Autodesk Inventor part; units mm, degrees
ref_plane "Work Plane1" through (0, 0, 0) normal (0, 0, 1) x (1, 0, 0)
ref_plane "YZ Plane" through (0, 0, 0) normal (1, 0, 0) x (0, 1, 0)
ref_plane "XZ Plane" through (0, 0, 0) normal (0, 1, 0) x (-1, 0, 0)
ref_plane "Work Plane1" through (0, 0, 0) normal (0, 0, 1) x (1, 0, 0)
sketch "Sketch1" plane through (0, 0, 0) normal (0, 0, 1) x (1, 0, 0)
  arc A0 (535, 222.5775) -> (565, 252.5775) centre (535, 252.5775) ccw
  line L0 (535, 222.5775) -> (295, 222.5775)
  arc A1 (265, 252.5775) -> (295, 222.5775) centre (295, 252.5775) ccw
  line L1 (265, 252.5775) -> (265, 402.5775)
  arc A2 (295, 432.5775) -> (265, 402.5775) centre (295, 402.5775) ccw
  line L2 (295, 432.5775) -> (535, 432.5775)
  arc A3 (565, 402.5775) -> (535, 432.5775) centre (535, 402.5775) ccw
  line L3 (565, 402.5775) -> (565, 252.5775)
  arc A4 (535, -104.9225) -> (565, -74.9225) centre (535, -74.9225) ccw
  line L4 (535, -104.9225) -> (295, -104.9225)
  arc A5 (265, -74.9225) -> (295, -104.9225) centre (295, -74.9225) ccw
  line L5 (265, -74.9225) -> (265, 75.0775)
  arc A6 (295, 105.0775) -> (265, 75.0775) centre (295, 75.0775) ccw
  line L6 (295, 105.0775) -> (535, 105.0775)
  arc A7 (565, 75.0775) -> (535, 105.0775) centre (535, 75.0775) ccw
  line L7 (565, 75.0775) -> (565, -74.9225)
  line L8 (565, -252.4225) -> (565, -402.4225)
  arc A8 (535, -432.4225) -> (565, -402.4225) centre (535, -402.4225) ccw
  line L9 (535, -432.4225) -> (295, -432.4225)
  arc A9 (265, -402.4225) -> (295, -432.4225) centre (295, -402.4225) ccw
  line L10 (265, -402.4225) -> (265, -252.4225)
  arc A10 (295, -222.4225) -> (265, -252.4225) centre (295, -252.4225) ccw
  line L11 (295, -222.4225) -> (535, -222.4225)
  arc A11 (565, -252.4225) -> (535, -222.4225) centre (535, -252.4225) ccw
  line L12 (-550, 375.7749) -> (-550, 187.5)
  arc A12 (-473.6326, 455.6923) -> (-550, 375.7749) centre (-470, 375.7749) ccw
  line L13 (229.0918, 487.6344) -> (-473.6326, 455.6923)
  arc A13 (250, 467.655) -> (229.0918, 487.6344) centre (230, 467.655) ccw
  line L14 (250, 187.5) -> (250, 467.655)
  arc A14 (230, 167.5) -> (250, 187.5) centre (230, 187.5) ccw
  line L15 (-530, 167.5) -> (230, 167.5)
  arc A15 (-550, 187.5) -> (-530, 167.5) centre (-530, 187.5) ccw
  arc A16 (250, -187.5) -> (230, -167.5) centre (230, -187.5) ccw
  line L16 (250, -467.655) -> (250, -187.5)
  arc A17 (229.0918, -487.6344) -> (250, -467.655) centre (230, -467.655) ccw
  line L17 (-473.6326, -455.6923) -> (229.0918, -487.6344)
  arc A18 (-550, -375.7749) -> (-473.6326, -455.6923) centre (-470, -375.7749) ccw
  line L18 (-550, -187.5) -> (-550, -375.7749)
  arc A19 (-530, -167.5) -> (-550, -187.5) centre (-530, -187.5) ccw
  line L19 (230, -167.5) -> (-530, -167.5)
  line L20 (-550, 137.5) -> (-550, -137.5)
  arc A20 (-530, 157.5) -> (-550, 137.5) centre (-530, 137.5) ccw
  line L21 (230, 157.5) -> (-530, 157.5)
  arc A21 (250, 137.5) -> (230, 157.5) centre (230, 137.5) ccw
  line L22 (250, -137.5) -> (250, 137.5)
  arc A22 (230, -157.5) -> (250, -137.5) centre (230, -137.5) ccw
  line L23 (-530, -157.5) -> (230, -157.5)
  arc A23 (-550, -137.5) -> (-530, -157.5) centre (-530, -137.5) ccw
  line L24 (570.1484, 510) -> (570.1484, -510)
  line L25 (500.9086, 510) -> (570.1484, 510)
  line L26 (-474.4993, 465.6633) -> (500.9086, 510)
  arc A24 (-474.4993, 465.6633) -> (-559.5063, 385.1982) centre (-470, 375.7749) ccw
  line L27 (-570.7648, 375.1108) -> (-559.5063, 385.1982)
  line L28 (-600, 375.7749) -> (-570.7648, 375.1108)
  line L29 (-600, -375.7749) -> (-600, 375.7749)
  line L30 (-570.7648, -375.1108) -> (-600, -375.7749)
  line L31 (-559.5063, -385.1982) -> (-570.7648, -375.1108)
  arc A25 (-559.5063, -385.1982) -> (-474.4993, -465.6633) centre (-470, -375.7749) ccw
  line L32 (500.9086, -510) -> (-474.4993, -465.6633)
  line L33 (570.1484, -510) -> (500.9086, -510)
  line L34 (250, 498.5951) -> (250, -498.5951)
  point P0 (0, 0)
extrude "Plate1" add sketch "Sketch1" against normal blind 1.5 contours L34 L26 L25 L24 L33 L32 L16 L22 L14
equation "\"d0\" = Thickness"
equation "\"BendRadius\" = Thickness"
equation "\"BendReliefWidth\" = Thickness"
equation "\"BendReliefDepth\" = 0.5 * Thickness"
equation "\"CornerReliefSize\" = 4 * Thickness"
equation "\"MinimumRemnant\" = 2 * Thickness"
equation "\"TransitionRadius\" = BendRadius"
equation "\"JacobiRadiusSize\" = BendRadius"
equation "\"GapSize\" = Thickness"
properties part number "CARCASA_ALUM_5"
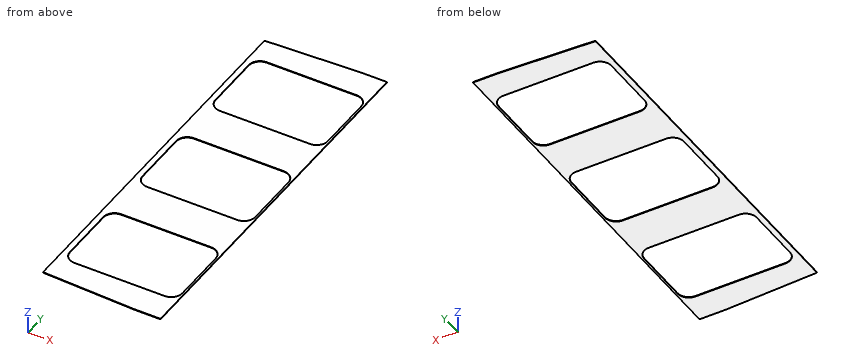
The listing builds one solid part. Answer for the finished solid, in the listing's coordinates (mm). Coordinates: 2 decimals unless noted, no trailing zeros. Write each loop counter-clockwise with the first axis right and the second up, starting at its lowest first coordinate (ties: lowest second). Pieces come first, ordered by that corner, then holes. Notation, with made-up numbers: (-19.5, -39.75) - (1.5, -39.75) arc R17 ccw to (1.5, -7.75) - close; hole circle Ø5 at (-13, 23.5). An arc over 180 degrees is marked (long way). Return JSON: item names as keys, results as strings. Group by question number.
1. A cutting plane is placed at D-D, the plane x = 415.5. Determine the outline of the cut face in (y, z).
2. Given pin 1 (0.8 mm diameter, centred on x = 464.5, z = -0.5, fed in from +Y); pin 2 (0.8 mm diameter, centred on x = 365.5, z = -0.5, fed in from -Y), each flat-ended and moving along its own axis, determine where each tip first touches the part or whether it passes through.
3. A cutting plane is placed at A-A, the plane z = -0.85. Give the number of separate pieces and of enclosed holes in the cut face, plus the area to 3 significant figures.
4. A cutting plane is placed at C-C, the plane x = 474.5. Determine the outline of the cut face in (y, z), plus the area to 3 significant figures.
5. A cutting plane is placed at B-B, the plane y = -36. Determine the outline of the cut face in (x, z).
6. Straight lines are drawn through the part: L1, parallel to Y at x = 502, z = -1.25; L2, parallel to Y at x = 537, z = -0.3; L3, parallel to X at y = -334.5, z = -0.3. For each, find the intervals that lie inside material, in ascending order.
Ans:
{
 "1": {"outline": "(-506.12, -1.5) - (-432.42, -1.5) - (-432.42, 0) - (-506.12, 0) - close; (-222.42, -1.5) - (-104.92, -1.5) - (-104.92, 0) - (-222.42, 0) - close; (105.08, -1.5) - (222.58, -1.5) - (222.58, 0) - (105.08, 0) - close; (432.58, -1.5) - (506.12, -1.5) - (506.12, 0) - (432.58, 0) - close"},
 "2": {"pin 1": "y = 508.36", "pin 2": "y = -503.86"},
 "3": {"separate pieces": "1", "enclosed holes": "3", "area": "137,000 mm²"},
 "4": {"outline": "(-508.8, -1.5) - (-432.42, -1.5) - (-432.42, 0) - (-508.8, 0) - close; (-222.42, -1.5) - (-104.92, -1.5) - (-104.92, 0) - (-222.42, 0) - close; (105.08, -1.5) - (222.58, -1.5) - (222.58, 0) - (105.08, 0) - close; (432.58, -1.5) - (508.8, -1.5) - (508.8, 0) - (432.58, 0) - close", "area": "581 mm²"},
 "5": {"outline": "(250, -1.5) - (265, -1.5) - (265, 0) - (250, 0) - close; (565, -1.5) - (570.15, -1.5) - (570.15, 0) - (565, 0) - close"},
 "6": {"L1": "-510 to -432.42, -222.42 to -104.92, 105.08 to 222.58, 432.58 to 510", "L2": "-510 to -432.36, -222.49 to -104.86, 105.01 to 222.64, 432.51 to 510", "L3": "250 to 265, 565 to 570.15"}
}
